```python
from build123d import *

# Parameters (mm, degrees)
BOSS_EXTRUDE1_DEPTH = 9
SKETCH2_R           = 1.5
CUT_EXTRUDE1_DEPTH  = 10


with BuildPart() as part:
    # Sketch1 → Boss-Extrude1 (new body)
    with BuildSketch(Plane.XY):
        with BuildLine():
            Line((2.05, 0), (10.242640687, 0))
            Line((10.242640687, 0), (10.242640687, 1.5))
            Line((10.242640687, 1.5), (4.242640687, 1.5))
            ThreePointArc((4.242640687, 1.5), (0, 4.5), (-4.242640687, 1.5))
            Line((-4.242640687, 1.5), (-10.242640687, 1.5))
            Line((-10.242640687, 1.5), (-10.242640687, 0))
            Line((-10.242640687, 0), (-2.05, 0))
            ThreePointArc((-2.05, 0), (0, 1.857268651), (2.05, 0))
        make_face()
    extrude(amount=BOSS_EXTRUDE1_DEPTH)

    # Sketch2 → Cut-Extrude1 (cut)
    with BuildSketch(Plane(origin=(0, 1.5, 0), x_dir=(1, 0, 0), z_dir=(0, 1, 0))):
        with Locations(Location((-7.242640687, -4.5, 0), (0, 0, 270))):
            Circle(SKETCH2_R)
        with Locations(Location((7.242640687, -4.5, 0), (0, 0, 270))):
            Circle(SKETCH2_R)
    extrude(amount=-CUT_EXTRUDE1_DEPTH, mode=Mode.SUBTRACT)


solid = part.part
```
Could you check a few things on this model? Use its own coordinates, in mm. A direction names the side the tool comes from. Coordinates: 2 decimals unless noted, no trailing zeros. Loops run counter-clockwise (first coordinate to the right, second up) from the corner with the lowest first, then second, coordinate; pieces in that order, holes last. Notation, with made-up numbers: M 82,9.25 L 129,9.25 A27 ccw 129,38.25 Z; hole C 66,19.5 d8. An arc over 180 degrees is marked long. Put each result on its own line as item: value. Start each with the question number.
(1) Suppose I cut it at D-D on x = 2.5. Please give me the cut outline in (y, z).
(2) I need wall thicknesses on line 1 (X direction, y = 1.15, z = 4.5); line 2 (X direction, y = 0.85, z = 1.25); line 3 (Y direction, x = -6.5, z = 2.75). Which ranges of each line are inside material? Lowest first, please. Write a range as from..to.
(3) Will these pins go through, and if not, where does the flat tip stop? P1, Ø2, axis at x = 7.5, z = 1.5, coming from the +Y side; P2, Ø2.5, axis at x = 7.24, z = 4.5, coming from the -Y side.
(4) Suppose I cut it at B-B on x = -6.75. Please give me the cut outline in (y, z), then the cut area to 3 significant figures.
(5) Suppose I cut it at C-C on z = 6.5. Please give me the cut outline in (x, y), then the cut area to 3 significant figures.
(6) Thinking about a two-plate mould opening in Z: for faces 1 (the face through (8.507, 0.76, 5.306)), 2 (the face through (-0.042, 1.857, 4.437)), 3 (the face through (-0.1, 2.3, 0)), which applies, pulls with the +Z half, pulls with the -Z half, needs draft (parallel to the pull), parting line crosses it, or undercut?
(7) For faces 4 (the face through (9, 1.5, 5)), 5 (the face through (-5.87, 1.5, 5.44)), 6 (the face through (0.1, 4.5, 4.4)), which set-ups out of +Z, -Z, +X, -X, +Y, -Y let a thin tool reach every point of the face, with its end or its side?
(8) Suppose I cut it at A-A on z = 4.5. Please give me the cut outline in (x, y).
Solutions:
1. outline: M 0,0 L 3.74,0 L 3.74,9 L 0,9 Z
2. line 1: x = -10.24..-8.74, -5.74..-1.55, 1.55..5.74, 8.74..10.24
2. line 2: x = -10.24..-1.77, 1.77..10.24
2. line 3: y = 0..1.5
3. P1: stops at y = 1.5
3. P2: passes through
4. outline: M 0,0 L 1.5,0 L 1.5,3.08 L 0,3.08 Z; M 0,5.92 L 1.5,5.92 L 1.5,9 L 0,9 Z
4. area: 9.25 mm2
5. outline: M -10.24,0 L -2.05,0 A2.06 cw 2.05,0 L 10.24,0 L 10.24,1.5 L 4.24,1.5 A4.5 ccw -4.24,1.5 L -10.24,1.5 Z
5. area: 43.5 mm2
6. face 1: undercut
6. face 2: needs draft
6. face 3: pulls with the -Z half
7. face 4: +Z, -Z, +X, +Y
7. face 5: +Z, -Z, -X, +Y
7. face 6: +Z, -Z, +Y
8. outline: M -10.24,0 L -8.74,0 L -8.74,1.5 L -10.24,1.5 Z; M -5.74,0 L -2.05,0 A2.06 cw 2.05,0 L 5.74,0 L 5.74,1.5 L 4.24,1.5 A4.5 ccw -4.24,1.5 L -5.74,1.5 Z; M 8.74,0 L 10.24,0 L 10.24,1.5 L 8.74,1.5 Z
